The listing builds one solid part. Answer for the finished solid, in the listing's coordinates (mm). Give positions to 0.01 mm unless a question says otherwise; leave off trailing zeros. Order: outer loops, then holes, each group sorted by start corner. A loop starts at its lowest first (then second) coordinate and runs counter-clockwise, first axis right, second up. Notation, with made-up numbers: (19.5, 89) - (38.5, 89) arc R25 cw to (38.5, 126) - close; hole circle Ø2 at (14.5, 86.5). An arc over 180 degrees is marked (long way). Write each question's results on one line, items separated by ' | '. Start each with the question number.
1. Determine the mould class of faces 1 (the face through (0.063, -3.987, 3.659)), 2 (the face through (6.885, 0.751, 2.071)), 3 (the face through (-9, 0, 1)) for opening direction X: released by +X, released by -X, zero draft, split by the parting line, or undercut.
2. A flat-ended cylindrical pin translates along its axis: pin 1 (1 mm diameter, centred on y = -2, z = 2.5, fed in from +X). Find the tip coordinate at first contact, or state that the pin passes through.
3. Section C-C (y = 0) is taken. State how many separate pieces and enclosed holes the cut face has, and give its area (3 significant figures).
4. Section D-D (x = 1.75) is taken. Give the vertices of the cut face in (y, z).
5. Section B-B (z = 2.15) is taken. Give the vertices of the cut face in (x, y).
6. Find the intervals of material crossed by L1, parallel to X at y = -0.25, z = 3.5; L2, parallel to Y at x = 4.5, z = 1.95; L3, parallel to Y at x = 3, z = 0.25, in increasing order.
7. Section A-A (x = -3) is taken. Give the vertices of the cut face in (y, z), and give its area (3 significant figures).
from build123d import *

# Parameters (mm, degrees)
SKETCH_R  = 2.5
PAD_DEPTH = 4.2
FILLET_R  = 1.8


with BuildPart() as part:
    # Sketch → Pad (new body)
    with BuildSketch(Plane.XY):
        with BuildLine():
            ThreePointArc((-4.5, 4.5), (-9, -1.4e-05), (-4.499972, -4.5))
            Line((-4.499972, -4.5), (4.5, -4.5))
            ThreePointArc((4.5, -4.5), (9, 1.4e-05), (4.499972, 4.5))
            Line((-4.5, 4.5), (4.499972, 4.5))
        make_face()
        with Locations((-4.5, 0)):
            Circle(SKETCH_R, mode=Mode.SUBTRACT)
        with Locations((4.5, 0)):
            Circle(SKETCH_R, mode=Mode.SUBTRACT)
    extrude(amount=PAD_DEPTH)

    # Fillet
    fillet_edges = [part.edges().sort_by_distance(p)[0] for p in [
        (9, 1.4e-05, 4.2),
    ]]
    fillet(fillet_edges, radius=FILLET_R)


solid = part.part
Reported:
1) face 1: zero draft | face 2: undercut | face 3: released by -X
2) pin 1: x = 8.74
3) separate pieces: 3 | enclosed holes: 0 | area: 32.2 mm²
4) outline: (-4.5, 0) - (4.5, 0) - (4.5, 2.4) arc R1.8 ccw to (2.7, 4.2) - (-2.7, 4.2) arc R1.8 ccw to (-4.5, 2.4) - close
5) outline: (-4.5, -4.5) - (4.5, -4.5) arc R4.5 ccw to (4.5, 4.5) - (-4.5, 4.5) arc R4.5 ccw to start; hole circle Ø5 at (-4.5, 0); hole circle Ø5 at (4.5, 0)
6) L1: -8.62 to -6.99, -2.01 to 2.01, 6.99 to 8.62 | L2: -4.5 to -2.5, 2.5 to 4.5 | L3: -4.5 to -2, 2 to 4.5
7) outline: (-4.5, 0) - (-2, 0) - (-2, 4.2) - (-2.7, 4.2) arc R1.8 ccw to (-4.5, 2.4) - close; (2, 0) - (4.5, 0) - (4.5, 2.4) arc R1.8 ccw to (2.7, 4.2) - (2, 4.2) - close | area: 19.6 mm²
